The model under review builds one solid part; all positions refer to its coordinate system, in mm. A direction names the side the tool comes from. Round coordinates to 2 decimals unless told otherwise and drop trailing zeros. Loops run counter-clockwise (first coordinate to the right, second up) from the corner with the lowest first, then second, coordinate; pieces in that order, holes last. Notation, with made-up numbers: (63.25, -5.75) -> (115.25, -5.75) arc R23 cw to (115.25, 16.25) -> close; hole circle Ø10 at (33.5, 5). An arc over 180 degrees is marked (long way). Return JSON: item names as keys, results as strings. Group by question number.
```python
from build123d import *

# Parameters (mm, degrees)
SKETCH_1_R          = 5.75
SKETCH_1_R_2        = 1.75
EXTRUDE_1_DEPTH     = 7
SKETCH_1_20_R       = 3.1
CUT_EXTRUDE_1_DEPTH = 2.6
EXTRUDE_START       = 5
SKETCH_1_21_W       = 24
SKETCH_1_21_H       = 11.5
SKETCH_1_21_R       = 1.75
EXTRUDE_2_DEPTH     = 2
SKETCH_2_R          = 1.5
CUT_EXTRUDE_2_DEPTH = 15.214868976
FILLET_1_R          = 5


with BuildPart() as part:
    # 草图1 → 凸台-拉伸1 (new body)
    with BuildSketch(Plane(origin=(0, 0, 0), x_dir=(1, 0, 0), z_dir=(0, 1, 0))):
        with Locations(Location((0, 0, 0), (0, 0, 270))):
            Circle(SKETCH_1_R)
        with Locations(Location((0, 0, 0), (0, 0, 270))):
            Circle(SKETCH_1_R_2, mode=Mode.SUBTRACT)
    extrude(amount=EXTRUDE_1_DEPTH)

    # 草图1<20> → 切除-拉伸1 (cut)
    with BuildSketch(Plane(origin=(0, 0, 0), x_dir=(1, 0, 0), z_dir=(0, 1, 0))):
        with Locations(Location((0, 0, 0), (0, 0, 270))):
            Circle(SKETCH_1_20_R)
    extrude(amount=CUT_EXTRUDE_1_DEPTH, mode=Mode.SUBTRACT)

    # 草图1<21> → 凸台-拉伸2 (add)
    with BuildSketch(Plane(origin=(0, 0, 0), x_dir=(1, 0, 0), z_dir=(0, 1, 0)).offset(EXTRUDE_START)):
        Rectangle(SKETCH_1_21_W, SKETCH_1_21_H)
        with Locations(Location((0, 0, 0), (0, 0, 270))):
            Circle(SKETCH_1_21_R, mode=Mode.SUBTRACT)
    extrude(amount=EXTRUDE_2_DEPTH)

    # 草图2 → 切除-拉伸2 (cut, through all)
    with BuildSketch(Plane.XZ.offset(-5)):
        with Locations(Location((-9, 0, 0), (0, 0, 270))):
            Circle(SKETCH_2_R)
        with Locations(Location((9, 0, 0), (0, 0, 270))):
            Circle(SKETCH_2_R)
    extrude(amount=-CUT_EXTRUDE_2_DEPTH, mode=Mode.SUBTRACT)

    # 圆角1
    fillet_1_edges = [part.edges().sort_by_distance(p)[0] for p in [
        (12, 6, 5.75),
        (-12, 6, 5.75),
        (-12, 6, -5.75),
        (12, 6, -5.75),
    ]]
    fillet(fillet_1_edges, radius=FILLET_1_R)


solid = part.part
```
1. Draft analysis for pull direction Z (two halves, no side actions). For faces 3 (the face through (7.536, 5.986, 0.325)), 4 (the face through (-12, 6, 0)), 5 (the face through (-10.57, 6.01, 4.25)), 6 (the face through (10.5, 6.01, -4.32)), state which applies: pulls with the +Z half, pulls with the -Z half, needs draft (parallel to the pull), parting line crosses it, or undercut.
2. For P1, Ø3.5, axis at x = 9, z = 0, coming from the -Y side; P2, Ø1.5, axis at x = 5, y = 3.5, coming from the -Z side, all flat-tipped, find the tip position at first contact; note any pin that passes through.
3. We need section B-B, the plane y = 5.25. Write out the cut boundary in (x, z), then the cut area to 3 significant figures.
4. Tool access review of faces 1 (the face through (12, 6, 0)), 2 (the face through (4.85, 2.46, 3.09)): name each direction out of +Z, -Z, +X, -X, +Y, -Y from which nothing blocks a thin tool from reaching the whole face with its end or side.
5. We need section A-A, the plane z = 0. Write out the cut boundary in (x, y).
6. We need section C-C, the plane x = -9. Write out the cut boundary in (y, z), then the cut area to 3 significant figures.
7. Wall thickness on line 1 (X direction, y = 6.1, z = 0); line 2 (X direction, y = 1.9, z = 0); line 3 (X direction, y = 4.9, z = 0): over which ranges is each line inside the solid? List them lowest first.
8. We need section D-D, the plane z = 4.75. Write out the cut boundary in (x, y), then the cut area to 3 significant figures.
Check sheet entries:
{
 "1": {"face 3": "undercut", "face 4": "needs draft", "face 5": "pulls with the +Z half", "face 6": "pulls with the -Z half"},
 "2": {"P1": "stops at y = 5", "P2": "stops at z = -3.87"},
 "3": {"outline": "(-12, -0.75) arc R5 ccw to (-7, -5.75) -> (7, -5.75) arc R5 ccw to (12, -0.75) -> (12, 0.75) arc R5 ccw to (7, 5.75) -> (-7, 5.75) arc R5 ccw to (-12, 0.75) -> close; hole circle Ø3 at (-9, 0); hole circle Ø3.5 at (0, 0); hole circle Ø3 at (9, 0)", "area": "231 mm²"},
 "4": {"face 1": "+Z, -Z, +X, +Y, -Y", "face 2": "-Y"},
 "5": {"outline": "(-12, 5) -> (-10.5, 5) -> (-10.5, 7) -> (-12, 7) -> close; (-7.5, 5) -> (-5.75, 5) -> (-5.75, 0) -> (-3.1, 0) -> (-3.1, 2.6) -> (-1.75, 2.6) -> (-1.75, 7) -> (-7.5, 7) -> close; (1.75, 2.6) -> (3.1, 2.6) -> (3.1, 0) -> (5.75, 0) -> (5.75, 5) -> (7.5, 5) -> (7.5, 7) -> (1.75, 7) -> close; (10.5, 5) -> (12, 5) -> (12, 7) -> (10.5, 7) -> close"},
 "6": {"outline": "(5, -5.33) -> (7, -5.33) -> (7, -1.5) -> (5, -1.5) -> close; (5, 1.5) -> (7, 1.5) -> (7, 5.33) -> (5, 5.33) -> close", "area": "15.3 mm²"},
 "7": {"line 1": "x = -12 to -10.5, -7.5 to -1.75, 1.75 to 7.5, 10.5 to 12", "line 2": "x = -5.75 to -3.1, 3.1 to 5.75", "line 3": "x = -5.75 to -1.75, 1.75 to 5.75"},
 "8": {"outline": "(-10, 5) -> (-3.24, 5) -> (-3.24, 0) -> (3.24, 0) -> (3.24, 5) -> (10, 5) -> (10, 7) -> (-10, 7) -> close", "area": "72.4 mm²"}
}
